Check sheet for the modelled part. Datum: model origin and axes. Units: mm. A direction names the side the tool comes from. Round coordinates to 2 decimals unless told otherwise and drop trailing zeros. Write each loop counter-clockwise with the first axis right and the second up, starting at its lowest first coordinate (ties: lowest second). Pieces come first, ordered by that corner, then holes. Notation, with made-up numbers: M -33,15.5 L -4,15.5 A13 ccw -4,33.5 Z; hole C -13,47.25 d7. An arc over 180 degrees is marked long. One line per item, written item: value.
Autodesk Fusion 360 part; units mm, degrees
sketch "Sketch1" plane through (0, 0, 0) normal (0, 1, 0) x (1, 0, 0)
  circle A0 centre (0, 0) radius 10.75
  line L0 (-9.8524, 4.3003) -> (-3, 20)
  line L1 (-3, 20) -> (3, 20)
  line L2 (3, 20) -> (9.8524, 4.3003)
  line L3 (0, 0) -> (0, 20) construction
  line L4 (3, 20) -> (0.75, 70)
  line L5 (0.75, 70) -> (-0.75, 70)
  line L6 (-0.75, 70) -> (-3, 20)
  line L7 (0, 20) -> (0, 70) construction
  dimension "d1" = 21.5
  dimension "d6" = 6
  dimension "d7" = 20
  dimension "d8" = 90
  dimension "d14" = 90
  dimension "d15" = 1.5
  dimension "d16" = 70
extrude "Extrude1" add sketch "Sketch1" along normal blind 2
sketch "Sketch2" plane through (0, 2, 0) normal (0, 1, 0) x (-1, 0, 0)
  arc A0 (9.8524, -4.3003) -> (-9.8524, -4.3003) centre (0, 0) ccw
  circle A1 centre (0, 0) radius 7
  line L0 (-9.8524, -4.3003) -> (-3, -20)
  line L1 (3, -20) -> (9.8524, -4.3003)
  line L2 (0, 0) -> (0, -7) construction
  circle A2 centre (0, -7) radius 1.75
  circle A3 centre (7, 0) radius 1.75
  circle A4 centre (0, 7) radius 1.75
  circle A5 centre (-7, 0) radius 1.75
  line L3 (-3, -20) -> (-0.75, -70)
  line L4 (-0.75, -70) -> (0.75, -70)
  line L5 (0.75, -70) -> (3, -20)
  dimension "d5" = 14
  dimension "d9" = 3.5
  dimension "d11" = 360
extrude "Extrude2" cut sketch "Sketch2" against normal up to surface (2 mm away) contours A1 A3 | A1 A3 | A1 A4 | A1 A4 | A1 A2 | A1 A2 | A1 A5 | A1 A5
sketch "Sketch4" plane through (0, 2, 0) normal (0, 1, 0) x (-1, 0, 0)
  circle A0 centre (7, 0) radius 1.75
  circle A1 centre (0, 7) radius 1.75
  circle A2 centre (0, -7) radius 1.75
  circle A3 centre (-7, 0) radius 1.75
  line L0 (-3, -20) -> (-0.75, -70)
  line L1 (-0.75, -70) -> (0.75, -70)
  line L2 (0.75, -70) -> (3, -20)
  line L3 (3, -20) -> (9.8524, -4.3003)
  arc A4 (9.8524, -4.3003) -> (-9.8524, -4.3003) centre (0, 0) ccw
  line L4 (-9.8524, -4.3003) -> (-3, -20)
  circle A5 centre (0, 0) radius 10.75 construction
sketch "Sketch3" plane through (0, 0, 0) normal (1, 0, 0) x (0, 0, -1)
  line L0 (-1.75, 2) -> (1.75, 2)
  line L1 (-8.75, 2) -> (-5.25, 2)
  line L2 (5.25, 2) -> (8.75, 2)
  line L3 (-1.75, 2) -> (1.75, 2)
  line L4 (20, 2) -> (70, 2)
  line L5 (70, 2) -> (20, 2)
  line L6 (20, 2) -> (4.3003, 2)
  line L7 (4.3003, 2) -> (-10.75, 2)
  line L8 (4.3003, 2) -> (20, 2)
  line L9 (10.75, 2) -> (-10.75, 2)
  line L10 (20.75, 2) -> (19.25, 2)
  line L11 (19.25, 2) -> (19.25, 10)
  line L12 (19.25, 10) -> (20.75, 10)
  line L13 (20.75, 10) -> (20.75, 2)
  line L14 (20, 10) -> (20, 2) construction
  dimension "d17" = 1.5
  dimension "d18" = 8
extrude "Extrude3" add sketch "Sketch3" along normal up to surface end surface through (-9.8524, 0, -4.3003) normal (-0.916505, 0, -0.400024) offset 0
mirror "Mirror1" about plane through (0, 0, 0) normal (1, 0, 0) of "Extrude3"
sketch "Sketch5" plane through (0, 2, 0) normal (0, 1, 0) x (-1, 0, 0)
  line L0 (-2.6726, -20.75) -> (-3, -20)
  line L1 (-3, -20) -> (-0.75, -70)
  line L2 (-0.75, -70) -> (0.75, -70)
  line L3 (0.75, -70) -> (3, -20)
  line L4 (3, -20) -> (2.6726, -20.75)
  line L5 (2.6726, -20.75) -> (-2.6726, -20.75)
  line L6 (2.6726, -20.75) -> (3.3274, -19.25)
  line L7 (3.3274, -19.25) -> (-3.3274, -19.25)
  line L8 (-3.3274, -19.25) -> (-2.6726, -20.75)
  line L9 (-2.6726, -20.75) -> (2.6726, -20.75)
  line L10 (2.6726, -20.75) -> (2.9663, -20.75)
  line L11 (-2.6726, -20.75) -> (-2.9663, -20.75)
  line L12 (0.75, -70) -> (-0.75, -70)
  line L13 (-0.75, -70) -> (-0.75, -20.75)
  line L14 (-0.75, -20.75) -> (0.75, -20.75)
  line L15 (0.75, -20.75) -> (0.75, -70)
  circle A0 centre (7, 0) radius 1.75
  circle A1 centre (0, 7) radius 1.75
  circle A2 centre (0, -7) radius 1.75
  circle A3 centre (-7, 0) radius 1.75
  line L16 (-3.3274, -19.25) -> (3.3274, -19.25)
  line L17 (3.3274, -19.25) -> (9.8524, -4.3003)
  arc A4 (9.8524, -4.3003) -> (-9.8524, -4.3003) centre (0, 0) ccw
  line L18 (-9.8524, -4.3003) -> (-3.3274, -19.25)
  circle A5 centre (0, 0) radius 10.75
extrude "Extrude4" add sketch "Sketch5" along normal up to surface (8 mm away) contours L0 L1 L8 L11 | L2 L5 L9 L12 L13 L14 L15 | L7 L16 L17 L18 A5 | L3 L4 L6 L10
sketch "Sketch6" plane through (0, 0, 0) normal (1, 0, 0) x (0, 0, -1)
  line L0 (20, 10) -> (20, 0)
  line L1 (20, 0) -> (4.3003, 0)
  line L2 (4.3003, 0) -> (4.3003, 2)
  line L3 (4.3003, 2) -> (4.3003, 10)
  line L4 (4.3003, 10) -> (20, 10)
  line L5 (70, 0) -> (20, 0)
  line L6 (20, 0) -> (20, 10)
  line L7 (20, 10) -> (20.75, 10)
  line L8 (20.75, 10) -> (20.75, 2)
  line L9 (20.75, 2) -> (70, 2)
  line L10 (70, 2) -> (70, 0)
  line L11 (20.75, 10) -> (70, 10)
  line L12 (70, 10) -> (70, 2)
  line L13 (70, 2) -> (20.75, 2)
  line L14 (20.75, 2) -> (20.75, 10)
  line L15 (4.3003, 0) -> (-10.75, 0)
  line L16 (4.3003, 0) -> (4.3003, 2)
  line L17 (4.3003, 2) -> (-10.75, 2)
  line L18 (4.3003, 2) -> (4.3003, 0)
  line L19 (10.75, 10) -> (4.3003, 10)
  line L20 (4.3003, 10) -> (4.3003, 2)
  line L21 (10.75, 2) -> (4.3003, 2)
  line L22 (4.3003, 2) -> (4.3003, 10)
  line L23 (8.75, 0) -> (5.25, 0)
  line L24 (5.25, 2) -> (8.75, 2)
  line L25 (7, 2) -> (7, 4.5)
  line L26 (7, 4.5) -> (18, 10)
  point P0 (7, 2)
  dimension "d25" = 2.5
  dimension "d26" = 2
extrude "Extrude5" cut sketch "Sketch6" against normal through all contours L3 L4 L19 L20 L21 L22 L24 L25 L26
mirror "Mirror2" about plane through (0, 0, 0) normal (1, 0, 0) of "Extrude5"
sketch "Sketch7" plane through (0, 0, 0) normal (1, 0, 0) x (0, 0, -1)
  line L0 (70, 10) -> (20.75, 10)
  line L1 (20.75, 10) -> (20.75, 2)
  line L2 (20.75, 2) -> (70, 2)
  line L3 (70, 2) -> (70, 10)
  line L4 (20, 0) -> (70, 0)
  line L5 (70, 0) -> (70, 2)
  line L6 (70, 2) -> (20.75, 2)
  line L7 (20.75, 2) -> (20.75, 10)
  line L8 (20.75, 10) -> (20, 10)
  line L9 (20, 10) -> (20, 0)
  line L10 (70, 7.5) -> (62.5, 0)
  dimension "d30" = 2.5
  dimension "d31" = 45
extrude "Extrude6" cut sketch "Sketch7" along normal through all contours L2 L3 L6 L10 | L2 L4 L5 L6 L10
mirror "Mirror3" about plane through (0, 0, 0) normal (1, 0, 0) of "Extrude6"
chamfer "Chamfer1" distance 2 angle 45 6 edges at (0.75, 6, -20.75) (0.75, 2, -42.625) (1.8581, 2, -20.75) (-0.75, 6, -20.75) (-1.8581, 2, -20.75) (-0.75, 2, -42.625)
chamfer "Chamfer2" distance 0.5 angle 45 2 edges at (-0.75, 8.75, -70) (0.75, 8.75, -70)
sketch "Sketch8" plane through (0, 2, 0) normal (0, 1, 0) x (-1, 0, 0)
  circle A0 centre (0, -7) radius 1.75
  arc A1 (-8.1586, -7) -> (8.1586, -7) centre (0, 0) ccw
  line L0 (8.1586, -7) -> (8.6741, -7)
  line L1 (8.6741, -7) -> (9.8524, -4.3003)
  arc A2 (9.8524, -4.3003) -> (-9.8524, -4.3003) centre (0, 0) ccw
  line L2 (-9.8524, -4.3003) -> (-8.6741, -7)
  line L3 (-8.6741, -7) -> (-8.1586, -7)
  circle A3 centre (7, 0) radius 1.75
  circle A4 centre (0, 7) radius 1.75
  circle A5 centre (-7, 0) radius 1.75
  circle A6 centre (0, 0) radius 3
  dimension "d37" = 6
extrude "Extrude7" cut sketch "Sketch8" against normal up to surface (2 mm away) contours A6
equation "d14 = d8"
Q1. Access from +Z, -Z, +X, -X, +Y, -Y to the whole of each face (thin tool, end or side, straight path). Record for faces 1 (the cylindrical face through (-0.13, 3.67, -10.75)), 2 (the flat face through (0.75, 7, -46)), 3 (the flat face through (-0.75, 7, -46)).
Completed:
face 1: +Z, +Y
face 2: -Z, +X, +Y
face 3: -Z, -X, +Y
Q2. Draft check along X on faces 4 (the flat face through (2.24, 2, 2.24)), 5 (the flat face through (-1.7, 7, -21.8)), 6 (the flat face through (0, 8, -14)), 7 (the cylindrical face through (-8.669, 1.014, 0.526)). Enter one of: pulls with the +X half, pulls with the -X half, needs draft (parallel to the pull), parting line crosses it, or undercut.
Completed:
face 4: undercut
face 5: pulls with the -X half
face 6: needs draft
face 7: undercut
Q3. Sectioned sample at B-B on x = 7. Enter the section's corners in (y, z).
Completed:
outline: M 0,-10.84 L 6.42,-10.84 L 5.08,-8.16 L 2,-8.16 L 2,-1.75 L 0,-1.75 Z; M 0,1.75 L 2,1.75 L 2,8.16 L 0,8.16 Z
Q4. Scan lines: line 1 (Z direction, x = 0, y = 1.35); line 2 (Z direction, x = 0, y = 0.7); line 3 (X direction, y = 0.5, z = -7). Record each from-to range of solid material in increasing order. Write a range as [from, to].
Completed:
line 1: [-63.85, -8.75], [-5.25, -3], [3, 5.25], [8.75, 10.75]
line 2: [-63.2, -8.75], [-5.25, -3], [3, 5.25], [8.75, 10.75]
line 3: [-8.67, -1.75], [1.75, 8.67]
Q5. Sectioned sample at A-A on z = 0. Enter the section's corners in (x, y).
Completed:
outline: M -10.75,0 L -8.75,0 L -8.75,2 L -10.75,2 Z; M -5.25,0 L -3,0 L -3,2 L -5.25,2 Z; M 3,0 L 5.25,0 L 5.25,2 L 3,2 Z; M 8.75,0 L 10.75,0 L 10.75,2 L 8.75,2 Z
Q6. Sectioned sample at D-D on y = 5.25. Enter the section's corners in (x, z).
Completed:
outline: M -8.02,-8.5 L -3.33,-19.25 L -3,-20 L -2.97,-20.75 L -2.75,-20.75 L -0.75,-22.75 L -0.75,-67.75 L 0.75,-67.75 L 0.75,-22.75 L 2.75,-20.75 L 2.97,-20.75 L 3,-20 L 3.33,-19.25 L 8.02,-8.5 L 6.58,-8.5 A10.75 cw -6.58,-8.5 Z
Q7. Depth check by flat-ended pin: P1, Ø5, axis at y = 6, z = -36, coming from the +X side; P2, Ø1.5, axis at y = 2.5, z = -12.5, coming from the +X side; P3, Ø10, axis at x = -5, z = -62, coming from the -Y side; P4, Ø4, axis at x = 0, z = -7, coming from the +Y side. Enter the tip coordinate at first touch or a pass-through.
Completed:
P1: x = 1.25
P2: x = 6.6
P3: y = 0
P4: y = 2
Q8. Sectioned sample at C-C on z = -35.5. Enter the section's corners in (x, y).
Completed:
outline: M -2.3,0 L 2.3,0 L 2.3,2.45 L 0.75,4 L 0.75,10 L -0.75,10 L -0.75,4 L -2.3,2.45 Z
